CAD build for the part. Positions are in the model's coordinates, mm. A direction names the side the tool comes from. Round coordinates to 2 decimals unless told otherwise and drop trailing zeros. Loops run counter-clockwise (first coordinate to the right, second up) from the corner with the lowest first, then second, coordinate; pieces in that order, holes last. Notation, with made-up numbers: M 15.5,-36.75 L 49.5,-36.75 A5 ccw 49.5,-31.75 Z; hole C -32,-7 d1. An arc over 180 degrees is marked long. Use one line per item in the form item = value.
Autodesk Inventor part; units mm, degrees
ref_plane "YZ Plane" through (0, 0, 0) normal (1, 0, 0) x (0, 1, 0)
ref_plane "XZ Plane" through (0, 0, 0) normal (0, 1, 0) x (-1, 0, 0)
ref_plane "XY Plane" through (0, 0, 0) normal (0, 0, 1) x (1, 0, 0)
sketch "Sketch1" plane through (0, 0, 0) normal (1, 0, 0) x (0, 1, 0)
  arc A0 (0, -16.7132) -> (0, 16.7132) centre (0, 0) ccw
  arc A1 (-198.0104, 16.7132) -> (-198.0104, -16.7132) centre (-198.0104, 0) ccw
  line L0 (0, 16.7132) -> (-198.0104, 16.7132)
  line L1 (-198.0104, -16.7132) -> (0, -16.7132)
  arc A2 (-198.0104, 18.3007) -> (-198.0104, -18.3007) centre (-198.0104, 0) ccw
  line L2 (-198.0104, -18.3007) -> (0, -18.3007)
  arc A3 (0, -18.3007) -> (0, 18.3007) centre (0, 0) ccw
  line L3 (0, 18.3007) -> (-198.0104, 18.3007)
  dimension "d0" = 16.7132
  dimension "d1" = 198.0104
  dimension "d2" = 1.5875
extrude "Extrusion1" add sketch "Sketch1" along normal blind 9
properties part number "STANDIN,BELT,100T,HTD5mm" material "Nylon 6/6"
1. Probe line 1 along Z through (x, y) = (6.25, -138); line 2 along Y through (x, z) = (8.25, -7.5); line 3 along Z through (x, y) = (5.5, 3). List the from-to ranges inside material, lowest first. Write a range as from..to.
Completed:
line_1 = -18.3..-16.71, 16.71..18.3
line_2 = -214.7..-212.95, 14.94..16.69
line_3 = -18.05..-16.44, 16.44..18.05
2. Pull direction Z, two halves, no side cores. Call faces 1 (the face through (4.44, 16.71, 0.37)), 2 (the face through (4, -98, 18.301)), 3 (the face through (4, -100, -18.301)): +Z half, -Z half, draft (parallel to the pull), parting line (faces both ways), or undercut.
Completed:
face_1 = undercut
face_2 = +Z half
face_3 = -Z half
3. Cut at C-C on x = 6. Write the cut outline in (y, z), and give its area (3 significant figures).
Completed:
outline = M -198.01,-18.3 L 0,-18.3 A18.3 ccw 0,18.3 L -198.01,18.3 A18.3 ccw Z; hole M -198.01,-16.71 L 0,-16.71 A16.71 ccw 0,16.71 L -198.01,16.71 A16.71 ccw Z
area = 803 mm2
4. Cut at B-B on y = -14. Write the cut outline in (x, z).
Completed:
outline = M 0,-18.3 L 9,-18.3 L 9,-16.71 L 0,-16.71 Z; M 0,16.71 L 9,16.71 L 9,18.3 L 0,18.3 Z
5. Cut at A-A on z = 0. Write the cut outline in (x, y).
Completed:
outline = M 0,-216.31 L 9,-216.31 L 9,-214.72 L 0,-214.72 Z; M 0,16.71 L 9,16.71 L 9,18.3 L 0,18.3 Z
6. Drop flat-ended pins along their axis: P1, Ø12, axis at y = -90.5, z = 12, coming from the -X side; P2, Ø2, axis at x = 1, z = -13, coming from the -Y side; P3, Ø4, axis at y = -74.5, z = -14, coming from the +X side. Give the stop position or say it passes through.
Completed:
P1 = 0
P2 = -211.83
P3 = through
7. Tool access for faces 4 (the face through (4.44, -214.72, -0.37)), 5 (the face through (0, -100, -18)): list every direction of +Z, -Z, +X, -X, +Y, -Y with a clear straight run to the whole face (end or side of a thin tool).
Completed:
face_4 = +X, -X
face_5 = +Z, -Z, -X, +Y, -Y
